Drawing for the job (mm, zero at the part's lowest x, y, z). Round coordinates to 2 decimals unless told otherwise and drop trailing zeros. Loops run counter-clockwise (first coordinate to the right, second up) from the corner with the lowest first, then second, coordinate; pieces in that order, holes last. Notation, with made-up numbers: (86.25, -7) -> (139.25, -7) arc R20 cw to (139.25, -1) -> close; hole circle Ø7 at (13, -29.75). An arc over 180 degrees is marked (long way). Put each result on its own line as item: value. Start each with the question number.
Item 1: Flat gauge pins, fed straight in: pin 1 Ø1.5 at (x, y) = (3.5, 31.5) entering from +Z; pin 2 Ø3 at (y, z) = (9.5, 2) entering from -X; pin 3 Ø5 at (x, y) = (1.5, 15) entering from -Z. Where does each tip first touch, or does it go through?
Item 2: Cut at B-B, the plane z = 4.5. List the corners of the cut face in (x, y).
Item 3: Cut at A-A, the plane x = 4.5. List the corners of the cut face in (y, z), plus the area to 3 significant figures.
Item 4: Cut at C-C, the plane y = 7. List the corners of the cut face in (x, z), plus the area to 3 significant figures.
Item 5: Cut at D-D, the plane z = 1. List the corners of the cut face in (x, y).
Item 6: Drill centre lines: probe 1 along X at (y, z) = (6.75, 4.5); probe 2 along Z at (x, y) = (4, 32). Where is each one in solid material? Low to high. Write a range as [from, to].
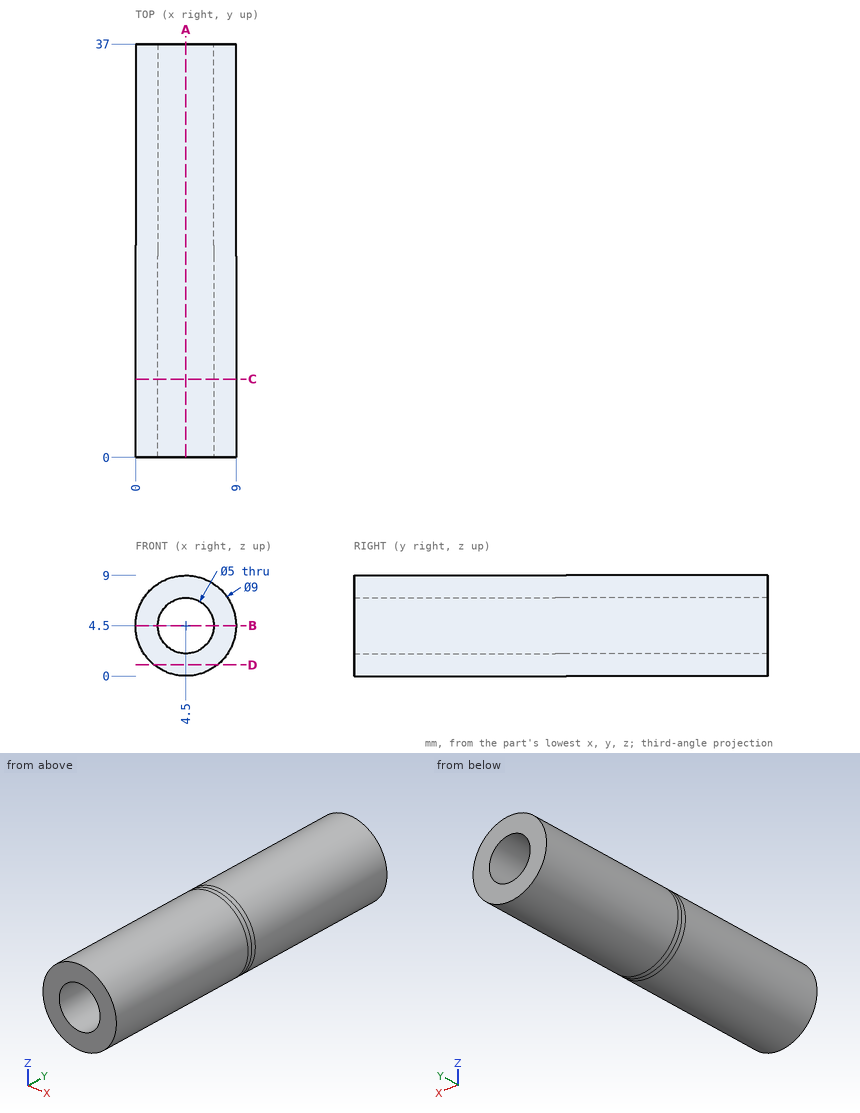
Reply:
1. pin 1: stops at z = 8.99
1. pin 2: stops at x = 0.11
1. pin 3: stops at z = 0.03
2. outline: (0, 0) -> (2, 0) -> (2, 37) -> (0, 37) -> close; (7, 0) -> (9, 0) -> (9, 37) -> (7, 37) -> close
3. outline: (0, 0) -> (37, 0) -> (37, 2) -> (0, 2) -> close; (0, 7) -> (37, 7) -> (37, 9) -> (0, 9) -> close
3. area: 148 mm^2
4. outline: circle Ø9 at (4.5, 4.5); hole circle Ø5 at (4.5, 4.5)
4. area: 44.0 mm^2
5. outline: (1.67, 0) -> (7.33, 0) -> (7.33, 37) -> (1.67, 37) -> close
6. probe 1: x = [0, 2], [7, 9]
6. probe 2: z = [0.03, 2.05], [6.95, 8.97]
